Can you work these out from the model? Positions are in its coordinate system, mm. Round coordinates to 2 decimals unless told otherwise and drop trailing zeros. Write each loop counter-clockwise with the first axis right and the second up, starting at its lowest first coordinate (ties: lowest second). Pieces come first, ordered by that corner, then holes. Notation, with made-up numbers: (48, 56.25) -> (93, 56.25) arc R18 cw to (93, 71.25) -> close; hole circle Ø10 at (-28, 53.5). An arc over 180 degrees is marked (long way). Write item = value, one per line. Start each with the question number.
1) I'm going to push flat-ended pins straight in: pin 1 (6 mm diameter, centred on x = 48.5, z = -27, fed in from +Y); pin 2 (3 mm diameter, centred on x = -17.3, z = -52.9, fed in from -Y); pin 3 (3 mm diameter, centred on x = 32.5, y = 11, fed in from +Z). Where does each tip first touch, or does it pass through?
2) If I drill on line 1 (X direction, y = 50.85, z = -52.9); line 2 (Z direction, x = 2.5, y = -6); line 3 (X direction, y = 5, z = 1), over which ranges is the centre line in solid material (lowest first)?
3) Imagine slicing it at A-A, the plane y = -17.8. Please give me the cut outline in (x, z).
4) Imagine slicing it at B-B, the plane y = -6. Please give me the cut outline in (x, z).
5) Thinking about a two-plate mould opening in Y: for faces 1 (the face through (41, 49.636, -53)), 2 (the face through (41, 51, -56.4)), 3 (the face through (41, 52.636, -53)), 4 (the face through (60.383, -20.188, 1.479)), which applies, +Y half, -Y half, draft (parallel to the pull), parting line (faces both ways), or undercut?
Autodesk Inventor part; units mm, degrees
ref_plane "YZ Plane" through (0, 0, 0) normal (1, 0, 0) x (0, 1, 0)
ref_plane "XZ Plane" through (0, 0, 0) normal (0, 1, 0) x (-1, 0, 0)
ref_plane "XY Plane" through (0, 0, 0) normal (0, 0, 1) x (1, 0, 0)
sketch "Esboço1" plane through (0, 0, 0) normal (0, 0, 1) x (1, 0, 0)
  line L0 (-21.8, -28.4) -> (-21.8, -58.8)
  line L1 (-16.1, -47.2) -> (-23.9, -47.2)
  line L2 (-26.1, 49.6356) -> (-29.1, 49.6356)
  line L3 (-21.8, -47.2) -> (101.8, -47.2)
  line L4 (101.8, -47.2) -> (101.8, 49.6356)
  line L5 (101.8, 49.6356) -> (-21.8, 49.6356)
  line L6 (-21.8, 49.6356) -> (-21.8, -47.2)
  line L7 (101.8, -28.4) -> (101.8, -58.8)
  circle A0 centre (27.2, -17.8) radius 7.95
  circle A1 centre (52.8, -17.8) radius 7.95
  circle A2 centre (40, -34.6) radius 1
  line L8 (-0.0154, 1.5) -> (75.5655, 1.5)
  line L9 (75.5655, 1.5) -> (106.1, 1.5)
  line L10 (-26.1, 1.5) -> (-0.0154, 1.5)
  point P0 (0, 0)
  point P1 (-21.8, 1.5)
  point P2 (101.8, 1.5)
  dimension "d0" = 0
extrude "Extrusão1" add sketch "Esboço1" along normal blind 3 contours L6 L10 L8 L9 L4 L3 L1 L0
sketch "Esboço2" plane through (101.8, -47.2, 0) normal (1, 0, 0) x (0, 0, -1)
  line L0 (0, 48.7) -> (0, 0)
  line L1 (0, 48.7) -> (-3, 48.7)
  line L2 (-3, 48.7) -> (-3, 55.7)
  line L3 (-3, 55.7) -> (0, 55.7)
  line L4 (0, 55.7) -> (0, 48.7)
  line L5 (16.4, 7.2) -> (16.4, 89.4875)
  line L6 (67.3088, 7.2) -> (16.4, 7.2)
  line L7 (57.4544, 17.0544) -> (67.3088, 7.2)
  arc A0 (56.4, 19.6) -> (57.4544, 17.0544) centre (60, 19.6) ccw
  line L8 (56.4, 35.6) -> (56.4, 19.6)
  arc A1 (63.6, 35.6) -> (56.4, 35.6) centre (60, 35.6) ccw
  line L9 (63.6, 21.0912) -> (63.6, 35.6)
  line L10 (77.4912, 7.2) -> (63.6, 21.0912)
  line L11 (109.9, 7.2) -> (77.4912, 7.2)
  line L12 (109.9, 77.4021) -> (109.9, 7.2)
  line L13 (53.4, 87.3646) -> (109.9, 77.4021)
  line L14 (53.4, 90.3646) -> (53.4, 87.3646)
  line L15 (56.4, 90.3646) -> (53.4, 90.3646)
  line L16 (56.4, 96.8356) -> (56.4, 90.3646)
  line L17 (49.4, 96.8356) -> (56.4, 96.8356)
  spline S0 degree 2 poles (16.4, 89.4875) (28.4788, 96.8356) (49.4, 96.8356) knots 0 0 0 1 1 1
  circle A2 centre (49.1, 41) radius 0.8
  line L18 (0, 55.7) -> (0, 96.8356) construction
  line L19 (0, 96.8356) -> (49.4, 96.8356) construction
  spline S1 degree 2 poles (0, 55.7) (0, 96.8356) (49.4, 96.8356) knots 1 1 1 2 2 2
  line L20 (49.4, 99.8356) -> (56.4, 99.8356)
  line L21 (56.4, 99.8356) -> (56.4, 96.8356)
  line L22 (56.4, 96.8356) -> (49.4, 96.8356)
  line L23 (49.4, 96.8356) -> (49.4, 99.8356)
  spline S2 degree 5 poles (-3, 55.7) (-3.0006, 59.6028) (-2.7317, 63.5042) (-2.1469, 67.3846) (-0.2515, 74.6) (3.2657, 81.1646) (5.3254, 84.0489) (10.316, 89.3567) (16.4783, 93.2583) (19.8737, 94.8743) (27.6563, 97.7143) (35.8292, 99.1582) (40.3418, 99.6246) (44.8718, 99.8357) (49.4, 99.8356) knots 0 0 0 0 0 0 0.249163 0.249163 0.249163 0.472611 0.472611 0.472611 0.710868 0.710868 0.710868 1 1 1 1 1 1
  point P0 (0, 47.2)
  point P1 (16.4, 89.4467)
  dimension "d3" = 7
extrude "Extrusão2" add sketch "Esboço2" against normal blind 123.6 contours L1 L2 L3 L4 | L3 S2 L23 S0 L5 S1 | L20 L21 L17 L23
sketch "Esboço3" plane through (0, 0, 3) normal (0, 0, 1) x (1, 0, 0)
  circle A0 centre (-17.8, 5.5) radius 1
  circle A1 centre (97.8, 5.5) radius 1
  point P0 (0, 0)
extrude "Extrusão3" cut sketch "Esboço3" against normal blind 6
sketch "Esboço4" plane through (101.8, 52.6356, -49.4) normal (0, 1, 0) x (1, 0, 0)
  circle A0 centre (-119.1, 3.5) radius 1
  circle A1 centre (-4.5, 3.5) radius 1
  point P0 (-101.8, -49.4)
extrude "Extrusão4" cut sketch "Esboço4" against normal blind 6
properties part number "frente recurva"
Reported:
q1.pin_1 = 50.71
q1.pin_2 = 49.64
q1.pin_3 = 2.99
q2.line_1 = -21.8 to -18.3, -16.3 to 96.3, 98.3 to 101.8
q2.line_2 = 0 to 3
q2.line_3 = -21.8 to -18.67, -16.93 to 96.93, 98.67 to 101.8
q3.outline = (-21.8, 0) -> (19.25, 0) -> (19.25, 3) -> (-21.8, 3) -> close; (35.15, 0) -> (44.85, 0) -> (44.85, 3) -> (35.15, 3) -> close; (60.75, 0) -> (101.8, 0) -> (101.8, 3) -> (60.75, 3) -> close
q4.outline = (-21.8, 0) -> (101.8, 0) -> (101.8, 3) -> (-21.8, 3) -> close
q5.face_1 = -Y half
q5.face_2 = draft
q5.face_3 = +Y half
q5.face_4 = undercut
